from build123d import *

# Parameters (mm, degrees)
BOSS_EXTRUDE1_DEPTH = 3


with BuildPart() as part:
    # Sketch1 → Boss-Extrude1 (new body)
    with BuildSketch(Plane.XY):
        Polygon((-0.65358299, 256.064124233), (0, 256.124180074), (-2.333831792, 256.338629089), (-6.241604492, 213.81064579), (-3.254189709, 213.536140934), (-7.189412895, 170.709416156), (-10.176827678, 170.983921012), (-14.084600378, 128.455937712), (-11.097185595, 128.181432856), (-15.03240878, 85.354708078), (-18.019823563, 85.629212934), (-21.927596263, 43.101229634), (-18.94018148, 42.826724778), (-22.875404666, 0), (22.875404666, 0), (25.862819449, 0.274504856), (21.955046749, 42.802488156), (18.967631966, 42.5279833), (15.03240878, 85.354708078), (18.019823563, 85.629212934), (14.112050863, 128.157196234), (11.12463608, 127.882691378), (7.189412895, 170.709416156), (10.176827678, 170.983921012), (6.269054978, 213.511904311), (3.281640195, 213.237399455), align=None)
    extrude(amount=BOSS_EXTRUDE1_DEPTH)


solid = part.part
Geometry: final body of the model. Coordinates: model frame, mm. A direction names the side the tool comes from. Round coordinates to 2 decimals unless told otherwise and drop trailing zeros. Order: outer loops, then holes, each group sorted by start corner. A loop starts at its lowest first (then second) coordinate and runs counter-clockwise, first axis right, second up. Notation, with made-up numbers: (18.25, -5) -> (60.25, -5) arc R15 cw to (60.25, -1) -> close; hole circle Ø11 at (0, -33.5). An arc over 180 degrees is marked (long way). Put each result on its own line as item: value. Start each with the question number.
Q1. Reachability of faces 1 (the flat face through (1, 101, 0)), 2 (the flat face through (-20.88, 21.71, 1.48)) from +Z, -Z, +X, -X, +Y, -Y: full face, straight path, thin tool, end or side. Return the list, or none.
Q2. Section A-A on z = 0.65. Return the cut outline in (x, y).
Q3. Line query: probe 1 along X at (y, z) = (112.5, 2.5); probe 2 along X at (y, z) = (211, 0.6); probe 3 along Y at (x, z) = (4.5, 0.65). Output: solid intervals per line, ascending.
Q4. First-contact query: pin 1 (1 mm diameter, centred on y = 181, z = 1.5, fed in from +X); pin 2 (1.5 mm diameter, centred on y = 54.5, z = 2, fed in from +X). Flat tips, straight axial feed; report the tip coordinate or a pass-through.
Q5. Section B-B on y = 111.5. Return the cut outline in (x, z), and give its area (3 significant figures).
Q6. Pull-direction query (Y, two-part tool) for faces 3 (the flat face through (17.028, 63.642, 1.479)), 4 (the flat face through (1, 101, 3)); classes: +Y half, -Y half, draft (parallel to the pull), parting line (faces both ways), or undercut.
Q7. Section C-C on y = 78. Return the cut outline in (x, z).
Ans:
1. face 1: -Z, +X, -X, +Y, -Y
1. face 2: +Z, -Z, -X
2. outline: (-22.88, 0) -> (22.88, 0) -> (25.86, 0.27) -> (21.96, 42.8) -> (18.97, 42.53) -> (15.03, 85.35) -> (18.02, 85.63) -> (14.11, 128.16) -> (11.12, 127.88) -> (7.19, 170.71) -> (10.18, 170.98) -> (6.27, 213.51) -> (3.28, 213.24) -> (-0.65, 256.06) -> (0, 256.12) -> (-2.33, 256.34) -> (-6.24, 213.81) -> (-3.25, 213.54) -> (-7.19, 170.71) -> (-10.18, 170.98) -> (-14.08, 128.46) -> (-11.1, 128.18) -> (-15.03, 85.35) -> (-18.02, 85.63) -> (-21.93, 43.1) -> (-18.94, 42.83) -> close
3. probe 1: x = -12.54 to 15.55
3. probe 2: x = -3.49 to 6.5
3. probe 3: y = 0 to 213.35
4. pin 1: stops at x = 9.3
4. pin 2: stops at x = 17.94
5. outline: (-12.63, 0) -> (15.64, 0) -> (15.64, 3) -> (-12.63, 3) -> close
5. area: 84.8 mm2
6. face 3: undercut
6. face 4: draft
7. outline: (-18.72, 0) -> (15.71, 0) -> (15.71, 3) -> (-18.72, 3) -> close
